Part print with two shaded views. Sizes in mm from the minimum x, y, z corner. A direction names the side the tool comes from. Coordinates: 2 decimals unless noted, no trailing zeros. Loops run counter-clockwise (first coordinate to the right, second up) from the corner with the lowest first, then second, coordinate; pieces in that order, holes last. Notation, with made-up numbers: (-15.75, 46) -> (-7.75, 46) arc R25 cw to (-7.75, 70) -> close; hole circle Ø4 at (-20.5, 61). An arc over 180 degrees is marked (long way). Write each question's results on one line, items separated by ' | '.
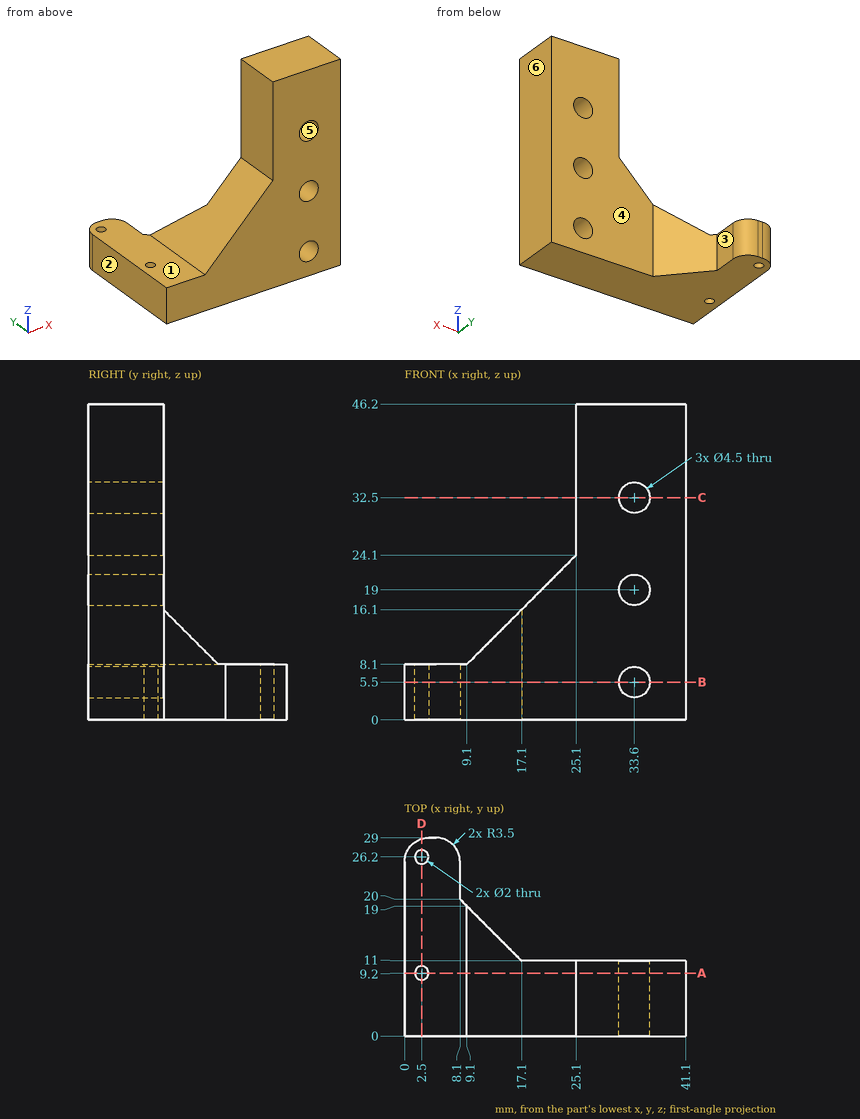
Q1. Cut at D-D on x = 2.5. Write the cut outline in (y, z).
Results are:
outline: (0, 0) -> (8.2, 0) -> (8.2, 8.1) -> (0, 8.1) -> close; (10.2, 0) -> (25.2, 0) -> (25.2, 8.1) -> (10.2, 8.1) -> close; (27.2, 0) -> (28.85, 0) -> (28.85, 8.1) -> (27.2, 8.1) -> close
Q2. Cut at B-B on z = 5.5. Write the cut outline in (x, y), and give its area (3 significant figures).
Results are:
outline: (0, 0) -> (31.35, 0) -> (31.35, 11) -> (17.1, 11) -> (8.1, 20) -> (8.1, 25.5) arc R3.5 ccw to (4.6, 29) -> (3.5, 29) arc R3.5 ccw to (0, 25.5) -> close; (35.85, 0) -> (41.1, 0) -> (41.1, 11) -> (35.85, 11) -> close; hole circle Ø2 at (2.5, 9.2); hole circle Ø2 at (2.5, 26.2) | area: 577 mm^2
Q3. Cut at A-A on y = 9.2. Write the cut outline in (x, z), and give its area (3 significant figures).
Results are:
outline: (0, 0) -> (1.5, 0) -> (1.5, 8.1) -> (0, 8.1) -> close; (3.5, 0) -> (41.1, 0) -> (41.1, 46.2) -> (25.1, 46.2) -> (25.1, 24.1) -> (9.1, 8.1) -> (3.5, 8.1) -> close; hole circle Ø4.5 at (33.6, 5.5); hole circle Ø4.5 at (33.6, 19); hole circle Ø4.5 at (33.6, 32.5) | area: 1,010 mm^2
Q4. Wall check: L1, parallel to X at y = 6.75, z = 5.5; L2, parallel to X at y = 3.75, z = 32.5; L3, parallel to Y at x = 2, z = 5. Give the ranges that are in metal, low to high. Write a range as from..to.
Results are:
L1: 0..31.35, 35.85..41.1 | L2: 25.1..31.35, 35.85..41.1 | L3: 0..8.33, 10.07..25.33, 27.07..28.66
Q5. Pull direction X, two halves, no side cores. Call the marked faces 4, 5 and 6: +X half, -X half, draft (parallel to the pull), parting line (faces both ways), or undercut.
Results are:
face 4: draft | face 5: undercut | face 6: +X half
Q6. Which spindle directions (+Z, -Z, +X, -X, +Y, -Y) get a long thin tool onto all of the face, cutting with end or side? Do the marked faces 1, 2 and 3. Say none if no direction does.
Results are:
face 1: +Z, -X, +Y, -Y | face 2: +Z, -Z, -X, +Y, -Y | face 3: +Z, -Z, +X, +Y
Q7. Drop flat-ended pins along their axis: pin 1 (10 mm diameter, centred on x = 3, y = 18.5, fed in from +Z); pin 2 (12 mm diameter, centred on x = 21, y = 10.5, fed in from -Z); pin 3 (9 mm diameter, centred on y = 5.5, z = 40, fed in from -X); pin 4 (6 mm diameter, centred on y = 24, z = 4.5, fed in from +X). Give the stop position or say it passes through.
Results are:
pin 1: z = 8.1 | pin 2: z = 0 | pin 3: x = 25.1 | pin 4: x = 8.1
Q8. Cut at C-C on z = 32.5. Write the cut outline in (x, y).
Results are:
outline: (25.1, 0) -> (31.35, 0) -> (31.35, 11) -> (25.1, 11) -> close; (35.85, 0) -> (41.1, 0) -> (41.1, 11) -> (35.85, 11) -> close
